Model file for the job. Use its own axes, mm. A direction names the side the tool comes from. Give positions to 0.01 mm unless a question says otherwise; leave off trailing zeros. Order: outer loops, then holes, each group sorted by start corner. A loop starts at its lowest first (then second) coordinate and runs counter-clockwise, first axis right, second up. Notation, with made-up numbers: (30.25, 75.25) - (80.25, 75.25) arc R22 ccw to (80.25, 101.25) - close; hole circle Ø6 at (4, 38.25). An arc over 180 degrees is marked (long way). Return JSON: item names as keys, results as strings. Group by question number.
from build123d import *

# Parameters (mm, degrees)
SKETCH_1_W      = 32.5
SKETCH_1_H      = 59.5
EXTRUDE_1_DEPTH = 42.4
EXTRUDE_2_DEPTH = 25
EXTRUDE_3_DEPTH = 1


with BuildPart() as part:
    # 草图1 → 拉伸1 (new body)
    with BuildSketch(Plane.XY):
        Rectangle(SKETCH_1_W, SKETCH_1_H)
    extrude(amount=EXTRUDE_1_DEPTH)

    # 草图2 → 拉伸2 (add)
    with BuildSketch(Plane.XY.offset(10)):
        with BuildLine():
            Line((-16.25, 20.932928605), (16.25, 20.932928605))
            ThreePointArc((16.25, 20.932928605), (26.5, 0), (16.25, -20.932928605))
            Line((16.25, -20.932928605), (-16.25, -20.932928605))
            ThreePointArc((-16.25, -20.932928605), (-26.5, 0), (-16.25, 20.932928605))
        make_face()
    extrude(amount=EXTRUDE_2_DEPTH)

    # 草图4 → 拉伸3 (add)
    # profile 1 of 2: a face of its own
    with BuildSketch(Plane.XY):
        with BuildLine():
            Line((-2, 44.25), (2, 44.25))
            ThreePointArc((2, 44.25), (6.242640687, 42.492640687), (8, 38.25))
            Line((8, 38.25), (8, 29.75))
            Line((8, 29.75), (-8, 29.75))
            Line((-8, 29.75), (-8, 38.25))
            ThreePointArc((-8, 38.25), (-6.242640687, 42.492640687), (-2, 44.25))
        make_face()
        with BuildLine():
            Line((-2.25, 38.25), (-2.25, 33.75))
            ThreePointArc((-2.25, 33.75), (0, 31.5), (2.25, 33.75))
            Line((2.25, 33.75), (2.25, 38.25))
            ThreePointArc((2.25, 38.25), (0, 40.5), (-2.25, 38.25))
        make_face(mode=Mode.SUBTRACT)
    # profile 2 of 2: a face of its own
    with BuildSketch(Plane.XY):
        with BuildLine():
            Line((-2, -44.25), (2, -44.25))
            ThreePointArc((2, -44.25), (6.242640687, -42.492640687), (8, -38.25))
            Line((8, -38.25), (8, -29.75))
            Line((8, -29.75), (-8, -29.75))
            Line((-8, -29.75), (-8, -38.25))
            ThreePointArc((-8, -38.25), (-6.242640687, -42.492640687), (-2, -44.25))
        make_face()
        with BuildLine():
            Line((2.25, -38.25), (2.25, -33.75))
            ThreePointArc((2.25, -33.75), (0, -31.5), (-2.25, -33.75))
            Line((-2.25, -33.75), (-2.25, -38.25))
            ThreePointArc((-2.25, -38.25), (0, -40.5), (2.25, -38.25))
        make_face(mode=Mode.SUBTRACT)
    extrude(amount=EXTRUDE_3_DEPTH)


solid = part.part
(1) Drill centre lines: L1, parallel to X at y = -25, z = 3; L2, parallel to Z at x = -18, y = 18; L3, parallel to Y at x = -4, z = 13. Where is each one in solid material? Low to high.
(2) Drop flat-ended pins along their axis: pin 1 Ø5 at (x, y) = (23.5, 2) entering from -Z; pin 2 Ø2 at (x, z) = (16, 19) entering from +Y; pin 3 Ø5 at (y, z) = (16, 8) entering from +X. Give the stop position or say it passes through.
(3) 3-axis set-ups, long thin cutter, end or side, ignore diameter. For faces 1 (the face through (20, 0, 35)), 2 (the face through (4, 37, 1)), 3 (the face through (-20, 0, 10)), 4 (the face through (0, -31.5, 0.5)): which of +Z, -Z, +X, -X, +Y, -Y reach the whole face in a straight line?
(4) Slice it at D-D (x = 14.5). Give the cut face in (y, z).
(5) Slice it at A-A (x = 0). Give the cut face in (y, z), and give its area (3 significant figures).
(6) Slice it at B-B (z = 17). Give the cut face in (x, y), and give its area (3 significant figures).
(7) Slice it at C-C (y = -1.5). Give the cut face in (x, z), and give its area (3 significant figures).
(8) Pull direction X, two halves, no side cores. Call faces 5 (the face through (20, 0, 10)), 6 (the face through (0, 40.5, 0.5)), 7 (the face through (-16.25, 0, 7)), 8 (the face through (16.25, 0, 7)): released by +X, released by -X, zero draft, split by the parting line, or undercut.
Result set:
{
 "1": {"L1": "x = -16.25 to 16.25", "L2": "z = 10 to 35", "L3": "y = -29.75 to 29.75"},
 "2": {"pin 1": "stops at z = 10", "pin 2": "stops at y = 29.75", "pin 3": "stops at x = 22.18"},
 "3": {"face 1": "+Z, +X, +Y, -Y", "face 2": "+Z, +X, -X, +Y", "face 3": "-Z, -X, +Y, -Y", "face 4": "+Z, -Z"},
 "4": {"outline": "(-29.75, 0) - (29.75, 0) - (29.75, 42.4) - (-29.75, 42.4) - close"},
 "5": {"outline": "(-44.25, 0) - (-40.5, 0) - (-40.5, 1) - (-44.25, 1) - close; (-31.5, 0) - (31.5, 0) - (31.5, 1) - (29.75, 1) - (29.75, 42.4) - (-29.75, 42.4) - (-29.75, 1) - (-31.5, 1) - close; (40.5, 0) - (44.25, 0) - (44.25, 1) - (40.5, 1) - close", "area": "2,530 mm²"},
 "6": {"outline": "(-16.25, -29.75) - (16.25, -29.75) - (16.25, -20.93) arc R26.5 ccw to (16.25, 20.93) - (16.25, 29.75) - (-16.25, 29.75) - (-16.25, 20.93) arc R26.5 ccw to (-16.25, -20.93) - close", "area": "2,530 mm²"},
 "7": {"outline": "(-26.46, 10) - (-16.25, 10) - (-16.25, 0) - (16.25, 0) - (16.25, 10) - (26.46, 10) - (26.46, 35) - (16.25, 35) - (16.25, 42.4) - (-16.25, 42.4) - (-16.25, 35) - (-26.46, 35) - close", "area": "1,890 mm²"},
 "8": {"face 5": "zero draft", "face 6": "undercut", "face 7": "released by -X", "face 8": "released by +X"}
}
